Work out the finished part from the listing and answer in its coordinate system (mm). A direction names the side the tool comes from. Coordinates: 2 decimals unless noted, no trailing zeros. Write each loop counter-clockwise with the first axis right and the second up, starting at its lowest first coordinate (ties: lowest second). Pieces come first, ordered by that corner, then holes. Notation, with made-up numbers: (66, 32) - (78, 32) arc R20 ccw to (78, 46) - close; hole circle Ø5 at (35.25, -35.75). An arc over 180 degrees is marked (long way). One line per item, written item: value.
Autodesk Inventor part; units mm, degrees
ref_plane "YZ Plane" through (0, 0, 0) normal (1, 0, 0) x (0, 1, 0)
ref_plane "XZ Plane" through (0, 0, 0) normal (0, 1, 0) x (-1, 0, 0)
ref_plane "XY Plane" through (0, 0, 0) normal (0, 0, 1) x (1, 0, 0)
sketch "Sketch1" plane through (0, 0, 0) normal (0, 1, 0) x (-1, 0, 0)
  circle A0 centre (5.65, 15.5) radius 1.6
  circle A1 centre (5.65, -15.5) radius 1.6
  arc A2 (7.65, 12.0359) -> (3.65, 18.9641) centre (5.65, 15.5) ccw
  arc A3 (3.65, -18.9641) -> (7.65, -12.0359) centre (5.65, -15.5) ccw
  line L0 (5.65, 15.5) -> (5.65, -15.5) construction
  circle A4 centre (-3.864, 8.4) radius 1.6
  circle A5 centre (-3.864, -8.4) radius 1.6
  line L1 (15.2493, 0) -> (-13.6973, 0)
  line L2 (0, -29.3497) -> (0, 29.3497)
  line L3 (-3.864, 8.4) -> (-3.864, -8.4) construction
  line L4 (-3.864, 11.8064) -> (-0.914, 10.1032)
  line L5 (-0.914, 10.1032) -> (-0.914, 6.6968)
  line L6 (-0.914, 6.6968) -> (-3.864, 4.9936)
  line L7 (-3.864, 4.9936) -> (-6.814, 6.6968)
  line L8 (-6.814, 6.6968) -> (-6.814, 10.1032)
  line L9 (-6.814, 10.1032) -> (-3.864, 11.8064)
  line L10 (-3.864, -4.9936) -> (-0.914, -6.6968)
  line L11 (-0.914, -6.6968) -> (-0.914, -10.1032)
  line L12 (-0.914, -10.1032) -> (-3.864, -11.8064)
  line L13 (-3.864, -11.8064) -> (-6.814, -10.1032)
  line L14 (-6.814, -10.1032) -> (-6.814, -6.6968)
  line L15 (-6.814, -6.6968) -> (-3.864, -4.9936)
  line L16 (-9.214, 9.805) -> (-9.214, -9.805)
  line L17 (-7.714, -12.4031) -> (3.65, -18.9641)
  line L18 (-7.714, 12.4031) -> (3.65, 18.9641)
  arc A6 (-7.714, 12.4031) -> (-9.214, 9.805) centre (-6.214, 9.805) ccw
  arc A7 (-9.214, -9.805) -> (-7.714, -12.4031) centre (-6.214, -9.805) ccw
  line L19 (7.65, 12.0359) -> (1.486, 8.4771)
  line L20 (1.486, 8.4771) -> (1.486, -8.4771)
  line L21 (1.486, -8.4771) -> (7.65, -12.0359)
  point P0 (0, 0)
  dimension "d0" = 31
  dimension "d2" = 3.2
  dimension "d3" = 3.2
  dimension "d6" = 8
  dimension "d7" = 8
  dimension "d32" = 16.8
  dimension "d33" = 15.5
  dimension "d34" = 8.4
  dimension "d35" = 5.65
  dimension "d36" = 3.864
  dimension "d37" = 3.2
  dimension "d38" = 3.2
  dimension "d39" = 5.9
  dimension "d40" = 5.9
  dimension "d41" = 2.4
  dimension "d42" = 3
  dimension "d45" = 2.4
extrude "Extrusion5" add sketch "Sketch1" along normal blind 3 contours L19 L20 L1 L2 L18 A2 | L2 L1 L16 A6 L18 | L20 L21 A3 L17 L2 L1 | L2 L17 A7 L16 L1 | L4 L5 L6 L7 L8 L9 | L10 L11 L12 L13 L14 L15
equation "\"d33\" = 0.5 * d0"
equation "\"d34\" = 0.5 * d32"
equation "\"d40\" = d39"
equation "\"d45\" = d41"
properties part number "TestMount"
Item 1: Section C-C, the plane x = -5 is taken. Determine the outline of the cut face in (y, z), then the cut area to 3 significant figures.
Evaluation:
outline: (0, -19.45) - (3, -19.45) - (3, -16.96) - (0, -16.96) - close; (0, -14.04) - (3, -14.04) - (3, -10.51) - (0, -10.51) - close; (0, 10.51) - (3, 10.51) - (3, 14.04) - (0, 14.04) - close; (0, 16.96) - (3, 16.96) - (3, 19.45) - (0, 19.45) - close
area: 36.1 mm2
Item 2: Section B-B, the plane y = 1.85 is taken. Determine the outline of the cut face in (x, z) (3 decimals).
Evaluation:
outline: (-7.65, -12.036) arc R4 ccw to (-3.65, -18.964) - (7.714, -12.403) arc R3 ccw to (9.214, -9.805) - (9.214, 9.805) arc R3 ccw to (7.714, 12.403) - (-3.65, 18.964) arc R4 ccw to (-7.65, 12.036) - (-1.486, 8.477) - (-1.486, -8.477) - close; hole circle Ø3.2 at (-5.65, -15.5); hole circle Ø3.2 at (-5.65, 15.5); hole circle Ø3.2 at (3.864, -8.4); hole circle Ø3.2 at (3.864, 8.4)
Item 3: Consider probe 1 along Z at (x, y) = (-6, 2.9); probe 2 along Z at (x, y) = (-5.75, 1.45); probe 3 along Z at (x, y) = (3.75, 2.9). Determine where each line is inside the solid, lowest interval first.
Evaluation:
probe 1: z = -19.48 to -17.06, -13.94 to -11.08, 11.08 to 13.94, 17.06 to 19.48
probe 2: z = -19.5 to -17.1, -13.9 to -10.94, 10.94 to 13.9, 17.1 to 19.5
probe 3: z = -14.69 to -10, -6.8 to 6.8, 10 to 14.69
Item 4: Given pin 1 (10 mm diameter, centred on x = 5.5, z = -12, fed in from -Y); pin 2 (0.9 mm diameter, centred on y = 1.5, z = 1, fed in from -X); pin 3 (1 mm diameter, centred on x = 5.5, y = 2.5, fed in from -Z), each flat-ended and moving along its own axis, determine where each tip first touches the part or whether it passes through.
Evaluation:
pin 1: stops at y = 0
pin 2: stops at x = -1.49
pin 3: stops at z = -13.97
Item 5: Section D-D, the plane z = 7.5 is taken. Determine the outline of the cut face in (x, y), then the cut area to 3 significant figures.
Evaluation:
outline: (-1.49, 0) - (2.54, 0) - (2.54, 3) - (-1.49, 3) - close; (5.19, 0) - (9.21, 0) - (9.21, 3) - (5.19, 3) - close
area: 24.2 mm2
Item 6: Which of the six approach directions +Z, -Z, +X, -X, +Y, -Y give full straight-line access (tool end or side, diameter ignored) to faces 4 (the face through (2.11, 1.48, 15.64)), 5 (the face through (-1.486, 1, 0))?
Evaluation:
face 4: +Z, +X, +Y, -Y
face 5: -X, +Y, -Y
Item 7: Section A-A, the plane z = 15.5 is taken. Determine the outline of the cut face in (x, y).
Evaluation:
outline: (-9.65, 0) - (-7.25, 0) - (-7.25, 3) - (-9.65, 3) - close; (-4.05, 0) - (2.35, 0) - (2.35, 3) - (-4.05, 3) - close
Item 8: Determine the mould class of faces 1 (the face through (0, 0, 0)), 2 (the face through (-5.442, 1.479, 13.914)), 3 (the face through (2.11, 1.48, -15.64)) for opening direction X: +X half, -X half, draft (parallel to the pull), parting line (faces both ways), or undercut.
Evaluation:
face 1: draft
face 2: undercut
face 3: +X half
